Work out the finished part from the listing and answer in its coordinate system (mm). Face numbers are marked on the shaded views. A direction names the side the tool comes from. Round coordinates to 2 decimals unless told otherwise and drop trailing zeros. Write each loop counter-clockwise with the first axis right and the second up, starting at its lowest first coordinate (ties: lowest second). Pieces come first, ordered by that corner, then holes. Notation, with made-up numbers: (-16, 23.5) -> (12, 23.5) arc R19 cw to (12, 41.5) -> close; hole circle Ø7 at (54, 13). An arc over 180 degrees is marked (long way). One line per item, written item: value.
```python
from build123d import *

# Parameters (mm, degrees)
CUT_EXTRUDE1_START  = -4
CUT_EXTRUDE1_DEPTH  = 4
BOSS_EXTRUDE1_DEPTH = 14.5
BOSS_EXTRUDE2_DEPTH = 2


with BuildPart() as part:
    # Sketch1 → Revolve1 (revolve)
    with BuildSketch(Plane.XY, mode=Mode.PRIVATE) as revolve1_sk:
        with BuildLine():
            Line((0, 8), (2, 8))
            Line((2, 8), (2, 4))
            Line((2, 4), (2.75, 4))
            Line((2.75, 4), (2.75, 1.4))
            ThreePointArc((2.75, 1.4), (3.892639488, 1.299222121), (5, 1))
            Line((5, 1), (5, 0))
            Line((5, 0), (0, 0))
            Line((0, 0), (0, 8))
        make_face()
    revolve(revolve1_sk.sketch.rotate(Axis((0, 8, 0), (0, -1, 0)), 180), axis=Axis((0, 8, 0), (0, -1, 0)))

    # Sketch2 → Cut-Extrude1 (cut)
    with BuildSketch(Plane(origin=(0, 8, 0), x_dir=(1, 0, 0), z_dir=(0, 1, 0)).offset(CUT_EXTRUDE1_START)):
        with BuildLine():
            Line((-1.377497731, 1.45), (1.377497731, 1.45))
            ThreePointArc((1.377497731, 1.45), (0, 2), (-1.377497731, 1.45))
        make_face()
    extrude(amount=CUT_EXTRUDE1_DEPTH, mode=Mode.SUBTRACT)

    # Sketch3 → Boss-Extrude1 (add)
    with BuildSketch(Plane.XZ):
        with BuildLine():
            Line((-1.75, -2.75), (1.75, -2.75))
            ThreePointArc((1.75, -2.75), (2.457106781, -2.457106781), (2.75, -1.75))
            Line((2.75, -1.75), (2.75, 1.75))
            ThreePointArc((2.75, 1.75), (2.457106781, 2.457106781), (1.75, 2.75))
            Line((1.75, 2.75), (-1.75, 2.75))
            ThreePointArc((-1.75, 2.75), (-2.457106781, 2.457106781), (-2.75, 1.75))
            Line((-2.75, 1.75), (-2.75, -1.75))
            ThreePointArc((-2.75, -1.75), (-2.457106781, -2.457106781), (-1.75, -2.75))
        make_face()
    extrude(amount=BOSS_EXTRUDE1_DEPTH)

    # Sketch5 → Boss-Extrude2 (add)
    with BuildSketch(Plane.XZ.offset(14.5)):
        with BuildLine():
            Line((1.3, -1.5), (-1.3, -1.5))
            ThreePointArc((-1.3, -1.5), (-1.441421356, -1.441421356), (-1.5, -1.3))
            Line((-1.5, -1.3), (-1.5, 1.3))
            ThreePointArc((-1.5, 1.3), (-1.441421356, 1.441421356), (-1.3, 1.5))
            Line((-1.3, 1.5), (1.3, 1.5))
            ThreePointArc((1.3, 1.5), (1.441421356, 1.441421356), (1.5, 1.3))
            Line((1.5, 1.3), (1.5, -1.3))
            ThreePointArc((1.5, -1.3), (1.441421356, -1.441421356), (1.3, -1.5))
        make_face()
    extrude(amount=BOSS_EXTRUDE2_DEPTH)


solid = part.part
```
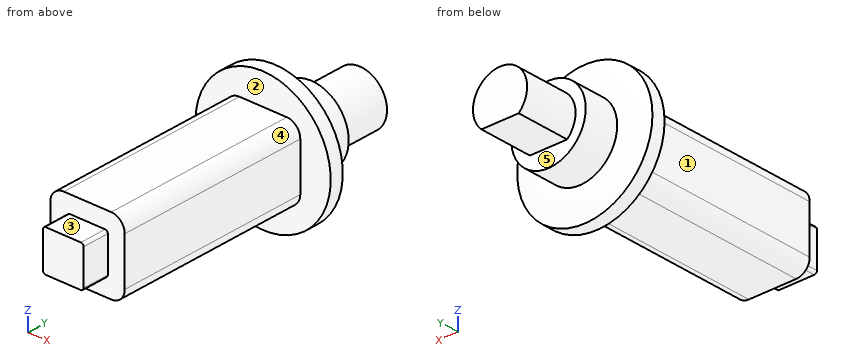
(1) Flat-ended cylindrical pins translate along their axes: pin 1 Ø1 at (y, z) = (-15.5, -0.5) entering from +X; pin 2 Ø1 at (x, y) = (0, -15.5) entering from +Z; pin 3 Ø4 at (x, y) = (-1, -5.5) entering from -Z; pin 4 Ø6 at (x, z) = (-1.5, -3.5) entering from +Y. Find the tip coordinate at first contact, or state that the pin passes through.
Reported:
pin 1: stops at x = 1.5
pin 2: stops at z = 1.5
pin 3: stops at z = -2.75
pin 4: stops at y = 8
(2) Find section B-B on y = 5.5. Give the vertices of the cut face in (x, z), plus the area to 3 significant figures.
Reported:
outline: (-1.38, -1.45) -> (1.38, -1.45) arc R2 ccw (long way) to start
area: 11.5 mm2
(3) Consider probe 1 along Z at (x, y) = (1.5, -12.75); probe 2 along Y at (x, z) = (1.5, 2.5). Determine where each line is inside the solid, lowest interval first.
Reported:
probe 1: z = -2.75 to 2.75
probe 2: y = -14.5 to 1.4
(4) A tool of negligible diameter and unlimited length cuts with its end or side. For the marked faces 1, 2, 3, 4 and 5, from which of +Z, -Z, +X, -X, +Y, -Y can it reach the whole face along a straight path? Write none if from no direction.
Reported:
face 1: +Z, -Z, -X, -Y
face 2: -Y
face 3: +Z, +X, -X, -Y
face 4: +Z, +X, -Y
face 5: +Y
(5) Find section A-A on y = -1.25. Give the vertices of the cut face in (x, z).
Reported:
outline: (-2.75, -1.75) arc R1 ccw to (-1.75, -2.75) -> (1.75, -2.75) arc R1 ccw to (2.75, -1.75) -> (2.75, 1.75) arc R1 ccw to (1.75, 2.75) -> (-1.75, 2.75) arc R1 ccw to (-2.75, 1.75) -> close
